Here's how the part is built. I have some questions about the finished solid (model axes, mm). A direction names the side the tool comes from. Round coordinates to 2 decimals unless told otherwise and drop trailing zeros. Write each loop counter-clockwise with the first axis right and the second up, starting at its lowest first coordinate (ties: lowest second). Pieces come first, ordered by that corner, then holes. Notation, with made-up numbers: (64.5, 76.25) -> (87.5, 76.25) arc R29 ccw to (87.5, 107.25) -> close; hole circle Ø2 at (46.5, 77.25). An arc over 180 degrees is marked (long way). Answer as CSV lines item,"result".
from build123d import *

# Parameters (mm, degrees)
SKETCH1_W           = 1.25
SKETCH1_H           = 5
BOSS_EXTRUDE1_DEPTH = 3.1
BOSS_EXTRUDE2_DEPTH = 9.5
BOSS_EXTRUDE3_DEPTH = 1.250000167
CUT_EXTRUDE1_DEPTH  = 0.7
CUT_EXTRUDE2_DEPTH  = 0.7
BOSS_EXTRUDE4_DEPTH = 0.6
SKETCH7_W           = 0.45
SKETCH7_H           = 1.7
CUT_EXTRUDE3_DEPTH  = 6.0000001
CUT_EXTRUDE4_REACH  = 13.55
SKETCH8_W           = 0.8
SKETCH8_H           = 1.25
SKETCH9_W           = 0.85
SKETCH9_H           = 1.25
CUT_EXTRUDE5_DEPTH  = 0.2
SKETCH10_W          = 0.05
SKETCH10_H          = 1.25
CUT_EXTRUDE6_DEPTH  = 0.2
CUT_EXTRUDE7_REACH  = 3.8
SKETCH12_W          = 0.6
SKETCH12_H          = 0.8
SKETCH13_W          = 0.45
SKETCH13_H          = 1.7
CUT_EXTRUDE8_DEPTH  = 6.0000001
SKETCH14_W          = 0.8
SKETCH14_H          = 1.25
CUT_EXTRUDE9_DEPTH  = 12.5500001
SKETCH15_W          = 0.85
SKETCH15_H          = 1.25
CUT_EXTRUDE10_DEPTH = 0.2
CUT_EXTRUDE11_REACH = 2.65
SKETCH17_W          = 0.1
SKETCH17_H          = 0.75
SKETCH18_W          = 1.5
SKETCH18_H          = 0.2
BOSS_EXTRUDE5_DEPTH = 0.4
CUT_EXTRUDE12_REACH = 2.65
SKETCH20_W          = 0.1
SKETCH20_H          = 0.75
CUT_EXTRUDE13_REACH = 2.65
SKETCH22_W          = 0.75
SKETCH22_H          = 0.1
SKETCH23_W          = 1.5
SKETCH23_H          = 0.2
BOSS_EXTRUDE6_DEPTH = 0.4
CUT_EXTRUDE14_REACH = 2.65
SKETCH25_W          = 0.75
SKETCH25_H          = 0.1
SKETCH26_W          = 0.05
SKETCH26_H          = 1.25
CUT_EXTRUDE15_DEPTH = 0.2
CUT_EXTRUDE16_REACH = 3.8
SKETCH28_W          = 0.6
SKETCH28_H          = 0.8
SKETCH29_W          = 0.25
SKETCH29_H          = 2.4
SKETCH30_W          = 0.25
SKETCH30_H          = 2.4
SKETCH31_W          = 0.25
SKETCH31_H          = 2.4
SKETCH32_W          = 0.25
SKETCH32_H          = 2.4
SKETCH33_W          = 0.25
SKETCH33_H          = 2.4
SKETCH34_W          = 0.25
SKETCH34_H          = 2.4
SKETCH35_W          = 0.25
SKETCH35_H          = 1.5
SKETCH36_W          = 0.25
SKETCH36_H          = 1.5
SKETCH37_W          = 0.25
SKETCH37_H          = 1.5
SKETCH38_W          = 0.25
SKETCH38_H          = 1.5
SKETCH39_W          = 0.25
SKETCH39_H          = 1.5
SKETCH40_W          = 0.25
SKETCH40_H          = 1.5


with BuildPart() as part:
    # Sketch1 → Boss-Extrude1 (new body)
    with BuildSketch(Plane.XY):
        with Locations((-5.375, 2.5)):
            Rectangle(SKETCH1_W, SKETCH1_H)
    extrude(amount=-BOSS_EXTRUDE1_DEPTH)

    # Sketch2 → Boss-Extrude2 (add)
    with BuildSketch(Plane(origin=(-4.75, 0, 0), x_dir=(0, 0, -1), z_dir=(1, 0, 0))):
        with BuildLine():
            Line((0, 5), (0.4, 5))
            Line((0.4, 5), (0.4, 1.9))
            Line((0.4, 1.9), (1.75, 1.9))
            Line((1.75, 1.9), (2.05, 1.6))
            Line((2.05, 1.6), (3.1, 1.6))
            add(Edge.make_bspline(
                [(3.1, 0), (3.1, 1.6)],
                knots=[0, 0, 0.32, 0.32], degree=1))
            Line((3.1, 0), (0, 0))
            Line((0, 0), (0, 5))
        make_face()
    extrude(amount=BOSS_EXTRUDE2_DEPTH)

    # Sketch3 → Boss-Extrude3 (add)
    with BuildSketch(Plane(origin=(4.75, 0, 0), x_dir=(0, 0, -1), z_dir=(1, 0, 0))):
        with BuildLine():
            Line((3.1, 0), (0, 0))
            Line((0, 0), (0, 5))
            Line((0, 5), (3.1, 5))
            add(Edge.make_bspline(
                [(3.1, 0), (3.1, 5)],
                knots=[0, 0, 1, 1], degree=1))
        make_face()
    extrude(amount=BOSS_EXTRUDE3_DEPTH)

    # Sketch4 → Cut-Extrude1 (cut)
    with BuildSketch(Plane(origin=(4.75, 0, 0), x_dir=(0, 0, -1), z_dir=(1, 0, 0))):
        Polygon((0.4, 1.9), (0.4, 3.2), (0, 3.2), (0, 0), (0.4, 0), align=None)
    extrude(amount=-CUT_EXTRUDE1_DEPTH, mode=Mode.SUBTRACT)

    # Sketch5 → Cut-Extrude2 (cut)
    with BuildSketch(Plane(origin=(-4.75, 0, 0), x_dir=(0, -1, 0), z_dir=(-1, 0, 0))):
        Polygon((-1.9, -0.4), (0, -0.4), (0, 0), (-3.2, 0), (-3.2, -0.4), align=None)
    extrude(amount=-CUT_EXTRUDE2_DEPTH, mode=Mode.SUBTRACT)

    # Sketch6 → Boss-Extrude4 (add)
    with BuildSketch(Plane(origin=(0, 0, -3.1), x_dir=(-1, 0, 0), z_dir=(0, 0, -1))):
        with BuildLine():
            add(Edge.make_bspline(
                [(6, 0), (-6, 0)],
                knots=[0, 0, 1, 1], degree=1))
            add(Edge.make_bspline(
                [(-6, 0), (-6, 5)],
                knots=[0, 0, 1, 1], degree=1))
            add(Edge.make_bspline(
                [(6, 5), (-6, 5)],
                knots=[0, 0, 1, 1], degree=1))
            add(Edge.make_bspline(
                [(6, 0), (6, 5)],
                knots=[0, 0, 1, 1], degree=1))
        make_face()
    extrude(amount=BOSS_EXTRUDE4_DEPTH)

    # Sketch7 → Cut-Extrude3 (cut, through all)
    with BuildSketch(Plane.XZ):
        with Locations((-5.775, -1.75)):
            Rectangle(SKETCH7_W, SKETCH7_H)
    extrude(amount=-CUT_EXTRUDE3_DEPTH, mode=Mode.SUBTRACT)

    # Sketch8 → Cut-Extrude4 (cut, up to next)
    with BuildSketch(Plane.ZY.offset(5.55), mode=Mode.PRIVATE) as cut_extrude4_sk1:
        with Locations((-1.35, 4.375)):
            Rectangle(SKETCH8_W, SKETCH8_H)
    cut_extrude4_tool1 = extrude(cut_extrude4_sk1.sketch, amount=-CUT_EXTRUDE4_REACH, mode=Mode.PRIVATE) & part.part
    add(cut_extrude4_tool1.solids().sort_by_distance((-5.55, 4.375, -1.35))[0], mode=Mode.SUBTRACT)

    # Sketch9 → Cut-Extrude5 (cut)
    with BuildSketch(Plane.ZY.offset(5.55)):
        with Locations((-2.175, 4.375)):
            Rectangle(SKETCH9_W, SKETCH9_H)
    extrude(amount=-CUT_EXTRUDE5_DEPTH, mode=Mode.SUBTRACT)

    # Sketch10 → Cut-Extrude6 (cut)
    with BuildSketch(Plane.ZY.offset(5.55)):
        with Locations((-0.925, 4.375)):
            Rectangle(SKETCH10_W, SKETCH10_H)
    extrude(amount=-CUT_EXTRUDE6_DEPTH, mode=Mode.SUBTRACT)

    # Sketch12 → Cut-Extrude7 (cut, up to next)
    with BuildSketch(Plane.XZ.offset(-3.2), mode=Mode.PRIVATE) as cut_extrude7_sk1:
        with Locations((-5.05, -1.35)):
            Rectangle(SKETCH12_W, SKETCH12_H)
    cut_extrude7_tool1 = extrude(cut_extrude7_sk1.sketch, amount=-CUT_EXTRUDE7_REACH, mode=Mode.PRIVATE) & part.part
    add(cut_extrude7_tool1.solids().sort_by_distance((-5.05, 3.2, -1.35))[0], mode=Mode.SUBTRACT)

    # Sketch13 → Cut-Extrude8 (cut, through all)
    with BuildSketch(Plane.XZ):
        with Locations((5.775, -1.75)):
            Rectangle(SKETCH13_W, SKETCH13_H)
    extrude(amount=-CUT_EXTRUDE8_DEPTH, mode=Mode.SUBTRACT)

    # Sketch14 → Cut-Extrude9 (cut, through all)
    with BuildSketch(Plane(origin=(5.55, 0, 0), x_dir=(0, 0, -1), z_dir=(1, 0, 0))):
        with Locations((1.35, 4.375)):
            Rectangle(SKETCH14_W, SKETCH14_H)
    extrude(amount=-CUT_EXTRUDE9_DEPTH, mode=Mode.SUBTRACT)

    # Sketch15 → Cut-Extrude10 (cut)
    with BuildSketch(Plane(origin=(5.55, 0, 0), x_dir=(0, 0, -1), z_dir=(1, 0, 0))):
        with Locations((2.175, 4.375)):
            Rectangle(SKETCH15_W, SKETCH15_H)
    extrude(amount=-CUT_EXTRUDE10_DEPTH, mode=Mode.SUBTRACT)

    # Sketch17 → Cut-Extrude11 (cut, up to next)
    with BuildSketch(Plane(origin=(-5.35, 0, 0), x_dir=(0, 0, -1), z_dir=(1, 0, 0)), mode=Mode.PRIVATE) as cut_extrude11_sk1:
        with Locations((0.95, 0.375)):
            Rectangle(SKETCH17_W, SKETCH17_H)
    cut_extrude11_tool1 = extrude(cut_extrude11_sk1.sketch, amount=-CUT_EXTRUDE11_REACH, mode=Mode.PRIVATE) & part.part
    add(cut_extrude11_tool1.solids().sort_by_distance((-5.35, 0.375, -0.95))[0], mode=Mode.SUBTRACT)

    # Sketch18 → Boss-Extrude5 (add)
    with BuildSketch(Plane.ZY.offset(5.55)):
        with Locations((-1.75, 0.1)):
            Rectangle(SKETCH18_W, SKETCH18_H)
    extrude(amount=BOSS_EXTRUDE5_DEPTH)

    # Sketch20 → Cut-Extrude12 (cut, up to next)
    with BuildSketch(Plane(origin=(-5.35, 0, 0), x_dir=(0, 0, -1), z_dir=(1, 0, 0)), mode=Mode.PRIVATE) as cut_extrude12_sk1:
        with Locations((2.55, 0.375)):
            Rectangle(SKETCH20_W, SKETCH20_H)
    cut_extrude12_tool1 = extrude(cut_extrude12_sk1.sketch, amount=-CUT_EXTRUDE12_REACH, mode=Mode.PRIVATE) & part.part
    add(cut_extrude12_tool1.solids().sort_by_distance((-5.35, 0.375, -2.55))[0], mode=Mode.SUBTRACT)

    # Sketch22 → Cut-Extrude13 (cut, up to next)
    with BuildSketch(Plane(origin=(5.35, 0, 0), x_dir=(0, -1, 0), z_dir=(-1, 0, 0)), mode=Mode.PRIVATE) as cut_extrude13_sk1:
        with Locations((-0.375, -2.55)):
            Rectangle(SKETCH22_W, SKETCH22_H)
    cut_extrude13_tool1 = extrude(cut_extrude13_sk1.sketch, amount=-CUT_EXTRUDE13_REACH, mode=Mode.PRIVATE) & part.part
    add(cut_extrude13_tool1.solids().sort_by_distance((5.35, 0.375, -2.55))[0], mode=Mode.SUBTRACT)

    # Sketch23 → Boss-Extrude6 (add)
    with BuildSketch(Plane(origin=(5.55, 0, 0), x_dir=(0, 0, -1), z_dir=(1, 0, 0))):
        with Locations((1.75, 0.1)):
            Rectangle(SKETCH23_W, SKETCH23_H)
    extrude(amount=BOSS_EXTRUDE6_DEPTH)

    # Sketch25 → Cut-Extrude14 (cut, up to next)
    with BuildSketch(Plane(origin=(5.35, 0, 0), x_dir=(0, -1, 0), z_dir=(-1, 0, 0)), mode=Mode.PRIVATE) as cut_extrude14_sk1:
        with Locations((-0.375, -0.95)):
            Rectangle(SKETCH25_W, SKETCH25_H)
    cut_extrude14_tool1 = extrude(cut_extrude14_sk1.sketch, amount=-CUT_EXTRUDE14_REACH, mode=Mode.PRIVATE) & part.part
    add(cut_extrude14_tool1.solids().sort_by_distance((5.35, 0.375, -0.95))[0], mode=Mode.SUBTRACT)

    # Sketch26 → Cut-Extrude15 (cut)
    with BuildSketch(Plane(origin=(5.55, 0, 0), x_dir=(0, 0, -1), z_dir=(1, 0, 0))):
        with Locations((0.925, 4.375)):
            Rectangle(SKETCH26_W, SKETCH26_H)
    extrude(amount=-CUT_EXTRUDE15_DEPTH, mode=Mode.SUBTRACT)

    # Sketch28 → Cut-Extrude16 (cut, up to next)
    with BuildSketch(Plane.XZ.offset(-3.2), mode=Mode.PRIVATE) as cut_extrude16_sk1:
        with Locations((5.05, -1.35)):
            Rectangle(SKETCH28_W, SKETCH28_H)
    cut_extrude16_tool1 = extrude(cut_extrude16_sk1.sketch, amount=-CUT_EXTRUDE16_REACH, mode=Mode.PRIVATE) & part.part
    add(cut_extrude16_tool1.solids().sort_by_distance((5.05, 3.2, -1.35))[0], mode=Mode.SUBTRACT)

    # Sketch29 → Revolve1 (revolve)
    with BuildSketch(Plane(origin=(0, 0, -1.3), x_dir=(-1, 0, 0), z_dir=(0, 0, -1))):
        with Locations((-3.875, 3.1)):
            Rectangle(SKETCH29_W, SKETCH29_H)
    revolve(axis=Axis((3.75, 1.9, -1.3), (0, 1, 0)))

    # Sketch30 → Revolve2 (revolve)
    with BuildSketch(Plane(origin=(0, 0, -1.3), x_dir=(-1, 0, 0), z_dir=(0, 0, -1))):
        with Locations((-2.375, 3.1)):
            Rectangle(SKETCH30_W, SKETCH30_H)
    revolve(axis=Axis((2.25, 1.9, -1.3), (0, 1, 0)))

    # Sketch31 → Revolve3 (revolve)
    with BuildSketch(Plane(origin=(0, 0, -1.3), x_dir=(-1, 0, 0), z_dir=(0, 0, -1))):
        with Locations((-0.875, 3.1)):
            Rectangle(SKETCH31_W, SKETCH31_H)
    revolve(axis=Axis((0.75, 1.9, -1.3), (0, 1, 0)))

    # Sketch32 → Revolve4 (revolve)
    with BuildSketch(Plane(origin=(0, 0, -1.3), x_dir=(-1, 0, 0), z_dir=(0, 0, -1))):
        with Locations((0.625, 3.1)):
            Rectangle(SKETCH32_W, SKETCH32_H)
    revolve(axis=Axis((-0.75, 1.9, -1.3), (0, 1, 0)))

    # Sketch33 → Revolve5 (revolve)
    with BuildSketch(Plane(origin=(0, 0, -1.3), x_dir=(-1, 0, 0), z_dir=(0, 0, -1))):
        with Locations((2.125, 3.1)):
            Rectangle(SKETCH33_W, SKETCH33_H)
    revolve(axis=Axis((-2.25, 1.9, -1.3), (0, 1, 0)))

    # Sketch34 → Revolve6 (revolve)
    with BuildSketch(Plane(origin=(0, 0, -1.3), x_dir=(-1, 0, 0), z_dir=(0, 0, -1))):
        with Locations((3.625, 3.1)):
            Rectangle(SKETCH34_W, SKETCH34_H)
    revolve(axis=Axis((-3.75, 1.9, -1.3), (0, 1, 0)))

    # Sketch35 → Revolve7 (revolve)
    with BuildSketch(Plane.XZ.offset(-0.25)):
        with Locations((3.875, -4.45)):
            Rectangle(SKETCH35_W, SKETCH35_H)
    revolve(axis=Axis((3.75, 0.25, -3.7), (0, 0, -1)))

    # Sketch36 → Revolve8 (revolve)
    with BuildSketch(Plane.XZ.offset(-0.25)):
        with Locations((2.375, -4.45)):
            Rectangle(SKETCH36_W, SKETCH36_H)
    revolve(axis=Axis((2.25, 0.25, -3.7), (0, 0, -1)))

    # Sketch37 → Revolve9 (revolve)
    with BuildSketch(Plane.XZ.offset(-0.25)):
        with Locations((0.875, -4.45)):
            Rectangle(SKETCH37_W, SKETCH37_H)
    revolve(axis=Axis((0.75, 0.25, -3.7), (0, 0, -1)))

    # Sketch38 → Revolve10 (revolve)
    with BuildSketch(Plane.XZ.offset(-0.25)):
        with Locations((-0.625, -4.45)):
            Rectangle(SKETCH38_W, SKETCH38_H)
    revolve(axis=Axis((-0.75, 0.25, -3.7), (0, 0, -1)))

    # Sketch39 → Revolve11 (revolve)
    with BuildSketch(Plane.XZ.offset(-0.25)):
        with Locations((-2.125, -4.45)):
            Rectangle(SKETCH39_W, SKETCH39_H)
    revolve(axis=Axis((-2.25, 0.25, -3.7), (0, 0, -1)))

    # Sketch40 → Revolve12 (revolve)
    with BuildSketch(Plane.XZ.offset(-0.25)):
        with Locations((-3.625, -4.45)):
            Rectangle(SKETCH40_W, SKETCH40_H)
    revolve(axis=Axis((-3.75, 0.25, -3.7), (0, 0, -1)))


solid = part.part
Item 1: Suppose I cut it at C-C, the plane y = 2.8. State how many separate pieces and enclosed holes the cut face has, then the cut area to 3 significant figures.
Results found:
separate pieces,"8"
enclosed holes,"0"
area,"17.8 mm²"
Item 2: For faces 1 (the flat face through (0, 1.9, -1)), 2 (the flat face through (4.75, 3, -2)), 3 (the flat face through (-5.35, 4, -2)), which set-ups out of +Z, -Z, +X, -X, +Y, -Y let a thin tool reach every point of the face, with its end or its side?
Results found:
face 1,"+Y"
face 2,"none"
face 3,"-X, +Y"
Item 3: Suppose I cut it at A-A, the plane z = -4.5. List the corners of the cut face in (x, y) for me, then the cut area to 3 significant figures.
Results found:
outline,"circle Ø0.5 at (-3.75, 0.25); circle Ø0.5 at (-2.25, 0.25); circle Ø0.5 at (-0.75, 0.25); circle Ø0.5 at (0.75, 0.25); circle Ø0.5 at (2.25, 0.25); circle Ø0.5 at (3.75, 0.25)"
area,"1.18 mm²"
Item 4: Suppose I cut it at B-B, the plane x = 5. List the corners of the cut face in (y, z) for me.
Results found:
outline,"(0, -3.7) -> (5, -3.7) -> (5, -1.75) -> (3.2, -1.75) -> (3.2, -0.95) -> (5, -0.95) -> (5, 0) -> (0, 0) -> close"
Item 5: I need wall thicknesses on L1, parallel to Z at x = -1, y = 4.7; L2, parallel to X at y = 2.25, z = -2.25; L3, parallel to X at y = 3.85, z = -1.8. Which ranges of each line are inside material? Lowest first, please.
Results found:
L1,"z = -3.7 to -3.1, -0.4 to 0"
L2,"x = -5.55 to -4.75, 4.75 to 5.55"
L3,"x = -5.35 to -4.75, 4.75 to 5.35"
Item 6: Suppose I cut it at D-D, the plane z = -2.25. List the corners of the cut face in (x, y) for me, then the cut area to 3 significant figures.
Results found:
outline,"(-5.95, 0) -> (5.95, 0) -> (5.95, 0.2) -> (5.55, 0.2) -> (5.55, 3.75) -> (5.35, 3.75) -> (5.35, 5) -> (4.75, 5) -> (4.75, 1.6) -> (-4.75, 1.6) -> (-4.75, 5) -> (-5.35, 5) -> (-5.35, 3.75) -> (-5.55, 3.75) -> (-5.55, 0.2) -> (-5.95, 0.2) -> close"
area,"22.9 mm²"
Item 7: If we mould it in two halves opening along Z, with no side actions, what happens to faces 4 (the flat face through (0, 3, -3.7)), 5 (the flat face through (5.55, 2, -2)), 6 (the flat face through (-0.1, 5, -0.2))? For each: pulls with the +Z half, pulls with the -Z half, needs draft (parallel to the pull), parting line crosses it, or undercut.
Results found:
face 4,"pulls with the -Z half"
face 5,"undercut"
face 6,"needs draft"
Item 8: Will this pin go through, and if not, where does the flat tip stop? pin 1 (0.7 mm diameter, centred on y = 4.5, z = -2, fed in from +X).
Results found:
pin 1,"stops at x = 5.35"
